For this review, take the finished solid that the model builds, in its own axes (mm). A direction names the side the tool comes from. Coordinates: 2 decimals unless noted, no trailing zeros. Write each loop counter-clockwise with the first axis right and the second up, starting at its lowest first coordinate (ties: lowest second). Pieces come first, ordered by that corner, then holes.
```python
from build123d import *

# Parameters (mm, degrees)
BOSS_EXTRUDE1_DEPTH  = 2.5
BOSS_EXTRUDE2_DEPTH  = 1.5
BOSS_EXTRUDE3_REACH  = 178.185
SKETCH4_W            = 4
SKETCH4_H            = 20
FILLET1_R            = 10
FILLET1_OF_MIRROR2_R = 10
SKETCH6_R            = 2.25
CUT_EXTRUDE2_DEPTH   = 130.700616807
SKETCH7_R            = 1.75
CUT_EXTRUDE3_DEPTH   = 130.700616807


with BuildPart() as part:
    # Sketch1 → Boss-Extrude1 (new body)
    with BuildSketch(Plane(origin=(0, 0, 0), x_dir=(0, 0, -1), z_dir=(1, 0, 0))):
        with BuildLine():
            Line((-62.5, -37.5), (-62.5, 37.5))
            ThreePointArc((-62.5, 37.5), (0, 100), (62.5, 37.5))
            Line((62.5, 37.5), (62.5, -37.5))
            ThreePointArc((62.5, -37.5), (0, -100), (-62.5, -37.5))
        make_face()
    extrude(amount=BOSS_EXTRUDE1_DEPTH)

    # Sketch2 → Boss-Extrude2 (add)
    with BuildSketch(Plane(origin=(2.5, 0, 0), x_dir=(0, 0, -1), z_dir=(1, 0, 0))):
        with BuildLine():
            Line((-60, 37.5), (-60, -37.5))
            ThreePointArc((-60, -37.5), (0, -97.5), (60, -37.5))
            Line((60, -37.5), (60, 37.5))
            ThreePointArc((60, 37.5), (0, 97.5), (-60, 37.5))
        make_face()
    extrude(amount=BOSS_EXTRUDE2_DEPTH)

    # Sketch4 → Boss-Extrude3 (add, up to next)
    with BuildSketch(Plane(origin=(0, 0, -82.5), x_dir=(-1, 0, 0), z_dir=(0, 0, -1)), mode=Mode.PRIVATE) as boss_extrude3_sk1:
        with Locations((-2, 45)):
            Rectangle(SKETCH4_W, SKETCH4_H)
    boss_extrude3_tool1 = extrude(boss_extrude3_sk1.sketch, amount=-BOSS_EXTRUDE3_REACH, mode=Mode.PRIVATE) - part.part
    # Sketch4 → Boss-Extrude3 (add, up to next)
    with BuildSketch(Plane(origin=(0, 0, -82.5), x_dir=(-1, 0, 0), z_dir=(0, 0, -1)), mode=Mode.PRIVATE) as boss_extrude3_sk2:
        with Locations((-2, -45)):
            Rectangle(SKETCH4_W, SKETCH4_H)
    boss_extrude3_tool2 = extrude(boss_extrude3_sk2.sketch, amount=-BOSS_EXTRUDE3_REACH, mode=Mode.PRIVATE) - part.part
    boss_extrude3_1 = boss_extrude3_tool1.solids().sort_by_distance((2, 45, -82.5))[0]
    add(boss_extrude3_1)
    boss_extrude3_2 = boss_extrude3_tool2.solids().sort_by_distance((2, -45, -82.5))[0]
    add(boss_extrude3_2)
    boss_extrude3 = boss_extrude3_1 + boss_extrude3_2  # Boss-Extrude3 as one shape, for the pattern or mirror that repeats it

    # Fillet1
    fillet1_edges = [part.edges().sort_by_distance(p)[0] for p in [
        (2, -55, -82.5),
        (2, -35, -82.5),
        (2, 35, -82.5),
        (2, 55, -82.5),
    ]]
    fillet(fillet1_edges, radius=FILLET1_R - 0.0001)  # a hair under: the kernel refuses the full size

    # Mirror2: Boss-Extrude3 across plane
    add(boss_extrude3.mirror(Plane(origin=(0, 0, 0), x_dir=(1, 0, 0), z_dir=(0, 0, -1))))

    # Fillet1 of Mirror2
    fillet1_of_mirror2_edges = [part.edges().sort_by_distance(p)[0] for p in [
        (2, -55, 82.5),
        (2, -35, 82.5),
        (2, 35, 82.5),
        (2, 55, 82.5),
    ]]
    fillet(fillet1_of_mirror2_edges, radius=FILLET1_OF_MIRROR2_R - 0.0001)  # a hair under: the kernel refuses the full size

    # Sketch6 → Cut-Extrude2 (cut, through all)
    with BuildSketch(Plane(origin=(4, 0, 0), x_dir=(0, 0, -1), z_dir=(1, 0, 0))):
        with Locations((-30, 40)):
            Circle(SKETCH6_R)
        with Locations(Location((30, 40, 0), (0, 0, 180))):
            Circle(SKETCH6_R)
        with Locations((30, -40)):
            Circle(SKETCH6_R)
        with Locations(Location((-30, -40, 0), (0, 0, 180))):
            Circle(SKETCH6_R)
    extrude(amount=-CUT_EXTRUDE2_DEPTH, mode=Mode.SUBTRACT)

    # Sketch7 → Cut-Extrude3 (cut, through all)
    with BuildSketch(Plane(origin=(4, 0, 0), x_dir=(0, 0, -1), z_dir=(1, 0, 0))):
        with Locations((0, 86.58)):
            Circle(SKETCH7_R)
        with Locations((49.3, 37.5)):
            Circle(SKETCH7_R)
        with Locations(Location((-49.3, 37.5, 0), (0, 0, 180))):
            Circle(SKETCH7_R)
        with Locations(Location((49.3, -37.5, 0), (0, 0, 180))):
            Circle(SKETCH7_R)
        with Locations(Location((0, -86.58, 0), (0, 0, 180))):
            Circle(SKETCH7_R)
        with Locations((-49.3, -37.5)):
            Circle(SKETCH7_R)
    extrude(amount=-CUT_EXTRUDE3_DEPTH, mode=Mode.SUBTRACT)


solid = part.part
```
1) Consider section A-A (z = -30). Give the boundary of the cut face in (x, y), then the cut area to 3 significant figures.
2) The part is to be moulded in two halves that separate along Y. For faces 1 (the face through (2, 35, 68)), 2 (the face through (1.23, 99.99, 1.13)), 3 (the face through (0, -1, 1)), say which applies: pulls with the +Y half, pulls with the -Y half, needs draft (parallel to the pull), parting line crosses it, or undercut.
3) For L1, parallel to Y at x = 2, z = 0; L2, parallel to Z at x = 3.55, y = 30; L3, parallel to Z at x = 2.25, y = -21, list the stretches that pass through material, from the lowest coordinate up.
4) Consider section C-C (y = -3). Give the boundary of the cut face in (x, z).
5) Consider section B-B (x = 3.2). Count the separate pieces of the cut face and the enclosed holes in it, then the cut area to 3 significant figures.
6) Tool access review of faces 4 (the face through (1.97, -38.01, -79.65)), 5 (the face through (3.24, -97.49, 1.07)), 6 (the face through (2.5, 98, 0)): name each direction out of +Z, -Z, +X, -X, +Y, -Y from which nothing blocks a thin tool from reaching the whole face with its end or side.
7) Clearance check with flat-ended pins moving along their axes: P1, Ø1.3, axis at y = 2.5, z = -61.5, coming from the +X side; P2, Ø1.5, axis at x = 3, y = -47, coming from the -Z side; P3, Ø1.2, axis at x = 0.5, y = 0, coming from the -Z side. State where each tip first meets the part, or that it passes through.
8) Consider section D-D (z = 23). Give the boundary of the cut face in (x, y), then the cut area to 3 significant figures.
Results:
1. outline: (0, -92.33) - (2.5, -92.33) - (2.5, -89.46) - (4, -89.46) - (4, -42.25) - (0, -42.25) - close; (0, -37.75) - (4, -37.75) - (4, 37.75) - (0, 37.75) - close; (0, 42.25) - (4, 42.25) - (4, 89.46) - (2.5, 89.46) - (2.5, 92.33) - (0, 92.33) - close
1. area: 694 mm2
2. face 1: undercut
2. face 2: pulls with the +Y half
2. face 3: needs draft
3. L1: y = -100 to -88.33, -84.83 to 84.83, 88.33 to 100
3. L2: z = -60 to 60
3. L3: z = -62.5 to 62.5
4. outline: (0, -62.5) - (2.5, -62.5) - (2.5, -60) - (4, -60) - (4, 60) - (2.5, 60) - (2.5, 62.5) - (0, 62.5) - close
5. separate pieces: 1
5. enclosed holes: 10
5. area: 21,900 mm2
6. face 4: -Z, +X, -X
6. face 5: +X, -Y
6. face 6: +X, +Y
7. P1: stops at x = 2.5
7. P2: stops at z = -82.42
7. P3: stops at z = -62.5
8. outline: (0, -95.61) - (2.5, -95.61) - (2.5, -92.92) - (4, -92.92) - (4, 92.92) - (2.5, 92.92) - (2.5, 95.61) - (0, 95.61) - close
8. area: 757 mm2
